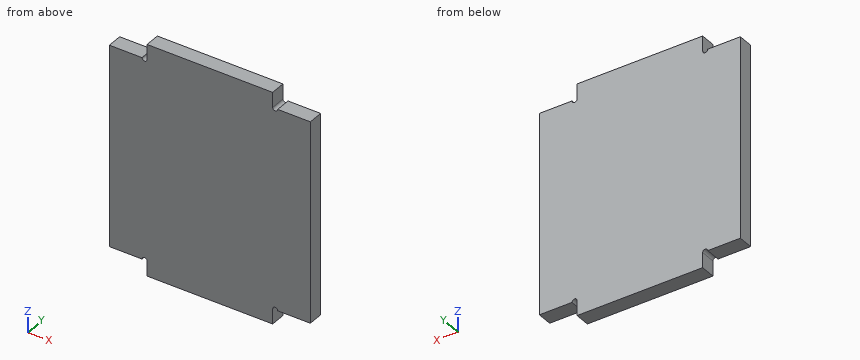
```python
from build123d import *

# Parameters (mm, degrees)
BOSS_EXTRUDE1_DEPTH = 3


with BuildPart() as part:
    # Sketch1 → Boss-Extrude1 (new body)
    with BuildSketch(Plane(origin=(0, 0, 0), x_dir=(1, 0, 0), z_dir=(0, 1, 0))):
        with BuildLine():
            Line((0, 0), (6.5, 0))
            ThreePointArc((6.5, 0), (7, 0.5), (7.5, 0))
            Line((7.5, 0), (7.5, -3))
            Line((7.5, -3), (32.5, -3))
            Line((32.5, -3), (32.5, 0))
            ThreePointArc((32.5, 0), (33, 0.5), (33.5, 0))
            Line((33.5, 0), (40, 0))
            Line((40, 0), (40, 40))
            Line((40, 40), (33.5, 40))
            ThreePointArc((33.5, 40), (33, 39.5), (32.5, 40))
            Line((32.5, 40), (32.5, 43))
            Line((32.5, 43), (7.5, 43))
            Line((7.5, 43), (7.5, 40))
            ThreePointArc((7.5, 40), (7, 39.5), (6.5, 40))
            Line((6.5, 40), (0, 40))
            Line((0, 40), (0, 0))
        make_face()
    extrude(amount=BOSS_EXTRUDE1_DEPTH)


solid = part.part
```
Source: CAD feature listing. Evaluate the final solid. Frame: model axes, mm. Round coordinates to 2 decimals unless told otherwise and drop trailing zeros. Order: outer loops, then holes, each group sorted by start corner. A loop starts at its lowest first (then second) coordinate and runs counter-clockwise, first axis right, second up. Notation, with made-up numbers: (25, 48) -> (48, 48) arc R29 cw to (48, 72) -> close; hole circle Ø11 at (9.5, 40.5). An arc over 180 degrees is marked (long way). One line per item, written item: value. Start each with the question number.
Q1. Section query A-A (y = 1.75). Return the cut outline in (x, z).
Q2. Section query B-B (x = 33). Return the cut outline in (y, z).
Q3. Pin query (flat end, axial travel): pin 1 (0.9 mm diameter, centred on y = 2, z = -41.5, fed in from +X); pin 2 (0.9 mm diameter, centred on y = 1.5, z = 2, fed in from -X); pin 3 (0.9 mm diameter, centred on x = 35.5, y = 2, fed in from -Z). Return the tip coordinate at first contact, or that it passes through.
Q4. Material intervals for probe 1 along Z at (x, y) = (33, 1.35); probe 2 along X at (y, z) = (1.25, -40.5); probe 3 along Z at (x, y) = (38.5, 1.4), sorted ascending.
Findings below:
1. outline: (0, -40) -> (6.5, -40) arc R0.5 cw to (7.5, -40) -> (7.5, -43) -> (32.5, -43) -> (32.5, -40) arc R0.5 cw to (33.5, -40) -> (40, -40) -> (40, 0) -> (33.5, 0) arc R0.5 cw to (32.5, 0) -> (32.5, 3) -> (7.5, 3) -> (7.5, 0) arc R0.5 cw to (6.5, 0) -> (0, 0) -> close
2. outline: (0, -39.5) -> (3, -39.5) -> (3, -0.5) -> (0, -0.5) -> close
3. pin 1: x = 32.5
3. pin 2: x = 7.5
3. pin 3: z = -40
4. probe 1: -39.5 to -0.5
4. probe 2: 7.5 to 32.5
4. probe 3: -40 to 0
